Here's how the part is built. I have some questions about the finished solid (model axes, mm). Face numbers are marked on the shaded views. A direction names the side the tool comes from. Round coordinates to 2 decimals unless told otherwise and drop trailing zeros. Loops run counter-clockwise (first coordinate to the right, second up) from the corner with the lowest first, then second, coordinate; pieces in that order, holes last. Notation, with made-up numbers: M -8.75,15 L 19.25,15 A22 cw 19.25,28 Z; hole C 45,63 d10. An arc over 180 degrees is marked long. One line per question, with ' | ' between items. Start each with the question number.
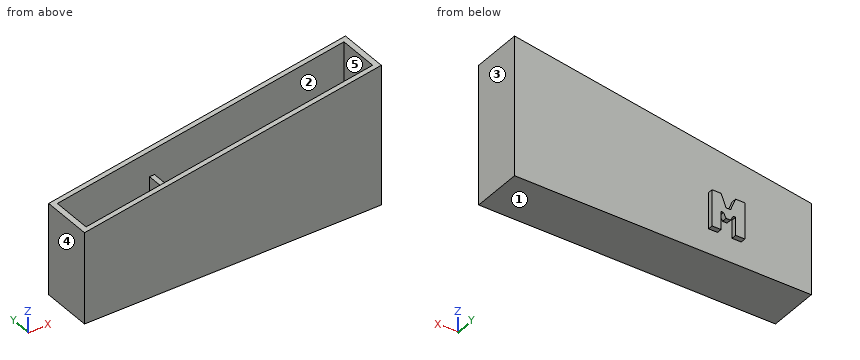
```python
from build123d import *

# Parameters (mm, degrees)
F1_DEPTH = 25.4
F2_T     = -2.54
F3_W     = 2.54
F3_H     = 20.32
F4_DEPTH = 38.1
F6_DEPTH = 2.54


with BuildPart() as f1:
    # F0 (on Front) → F1 (new body)
    with BuildSketch(Plane.XZ):
        Polygon((-66.060728, 15.077978), (-66.060728, -30.15408), (81.259272, -30.15408), (81.259272, 39.08381), align=None)
    extrude(amount=F1_DEPTH)

    # F2
    f2_openings = [f1.faces().sort_by_distance(p)[0] for p in [
        (7.599272, -12.7, 27.080894),
    ]]
    offset(amount=F2_T, openings=f2_openings)

    # F3 (on face) → F4 (join)
    with BuildSketch(Plane.XY.offset(-27.61408)):
        with Locations((31.729272, -12.7)):
            Rectangle(F3_W, F3_H)
        with Locations((-16.530728, -12.7)):
            Rectangle(F3_W, F3_H)
    extrude(amount=F4_DEPTH)

    # F5 (on Front) → F6 (join)
    with BuildSketch(Plane.XZ):
        Polygon((-26.697874, 0), (-31.276897, 0), (-31.276897, -17.934263), (-26.697874, -17.934263), (-26.697874, -8.967131), (-25.506107, -8.967131), (-24.200872, -11.420006), (-23.090161, -11.420006), (-21.97945, -11.420006), (-20.674216, -8.967131), (-19.482449, -8.967131), (-19.482449, -17.934263), (-15.020955, -17.934263), (-15.020955, 0), (-19.482449, 0), (-21.97945, -6.206409), (-24.200872, -6.206409), align=None)
    extrude(amount=-F6_DEPTH)


solid = f1.part
```
1) Imagine slicing it at A-A (z = -25). Write out the boundary of the cut face in (x, y), then the cut area to 3 significant figures.
2) I'm going to push flat-ended pins straight in: pin 1 Ø2 at (x, y) = (31.5, -12.5) entering from +Z; pin 2 Ø1.3 at (x, y) = (-26, 1) entering from -Z; pin 3 Ø0.8 at (y, z) = (1, -15.5) entering from +X; pin 4 Ø4 at (x, z) = (-31, 23.5) entering from -Y. Where does each tip first touch, or does it pass through?
3) For the marked faces 1 and 2, which set-ups out of +Z, -Z, +X, -X, +Y, -Y let a thin tool reach every point of the face, with its end or its side?
4) Imagine slicing it at C-C (y = -6.25). Write out the boundary of the cut face in (x, z).
5) Please list where these lines run through material, in increasing order: L1, parallel to X at y = -3.5, z = -3.5; L2, parallel to Y at x = 57, z = 13; L3, parallel to Z at x = -27, y = -5. Write a range as from..to.
6) Imagine slicing it at B-B (x = -42). Write out the boundary of the cut face in (y, z).
7) We'd pull the mould along X, two halves only. Please class the marked faces 3, 4 and 5: pulls with the +X half, pulls with the -X half, needs draft (parallel to the pull), parting line crosses it, or undercut.
8) Imagine slicing it at D-D (z = 21.5). Write out the boundary of the cut face in (x, y), then the cut area to 3 significant figures.
Results are:
1) outline: M -66.06,-25.4 L 81.26,-25.4 L 81.26,0 L -66.06,0 Z; hole M -63.52,-22.86 L -17.8,-22.86 L -17.8,-2.54 L -63.52,-2.54 Z; hole M -15.26,-22.86 L 30.46,-22.86 L 30.46,-2.54 L -15.26,-2.54 Z; hole M 33,-22.86 L 78.72,-22.86 L 78.72,-2.54 L 33,-2.54 Z | area: 955 mm²
2) pin 1: z = 10.49 | pin 2: z = -9.26 | pin 3: x = -15.02 | pin 4: through
3) face 1: -Z, +X, -X, +Y, -Y | face 2: +Z
4) outline: M -66.06,-30.15 L 81.26,-30.15 L 81.26,39.08 L 78.72,38.67 L 78.72,-27.61 L 33,-27.61 L 33,10.49 L 30.46,10.49 L 30.46,-27.61 L -15.26,-27.61 L -15.26,10.49 L -17.8,10.49 L -17.8,-27.61 L -63.52,-27.61 L -63.52,15.49 L -66.06,15.08 Z
5) L1: -66.06..-63.52, -17.8..-15.26, 30.46..33, 78.72..81.26 | L2: -25.4..-22.86, -2.54..0 | L3: -30.15..-27.61
6) outline: M -25.4,-30.15 L 0,-30.15 L 0,19 L -2.54,19 L -2.54,-27.61 L -22.86,-27.61 L -22.86,19 L -25.4,19 Z
7) face 3: pulls with the +X half | face 4: pulls with the -X half | face 5: undercut
8) outline: M -26.65,-25.4 L 81.26,-25.4 L 81.26,0 L -26.65,0 L -26.65,-2.54 L 78.72,-2.54 L 78.72,-22.86 L -26.65,-22.86 Z | area: 600 mm²
